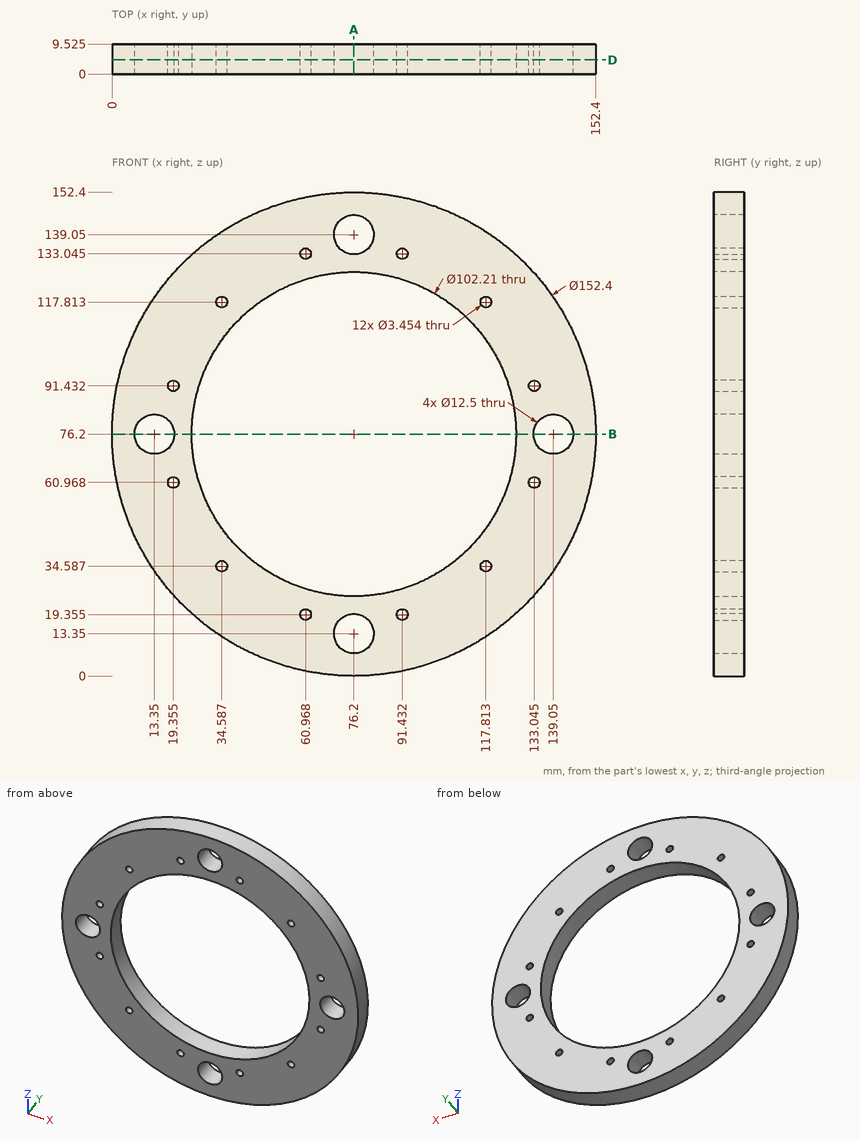
The drawing under review shows one solid part. Ordinate dimensions are in mm from its lowest x, y, z. Round coordinates to 2 decimals unless told otherwise and drop trailing zeros. Write each loop counter-clockwise with the first axis right and the second up, starting at its lowest first coordinate (ties: lowest second). Pieces come first, ordered by that corner, then holes. Notation, with made-up numbers: M 25,-16 L 66,-16 A31 cw 66,8 Z; hole C 16.5,9.5 d2. An arc over 180 degrees is marked long. One line per item, written item: value. Start each with the question number.
(1) We need section A-A (x = 76.2). Give the boundary of the cut face in (y, z) (1 decimal), and give its area (3 significant figures).
(2) Insertion check: pin 1 (1.5 mm diameter, centred on x = 119.5, y = 6.5, fed in from +Z); pin 2 (1 mm diameter, centred on x = 17, y = 5.5, fed in from +Z); pin 3 (5 mm diameter, centred on x = 57.5, y = 5, fed in from +Z). Each pin has a flat end and moves straight along its axis. Give the tip position at first contact, or say it passes through.
(3) We need section D-D (y = 4.5). Count the separate pieces of the cut face and the enclosed holes in it, and give its area (3 significant figures).
(4) Wall thickness on line 1 (X direction, y = 3.25, z = 76.2) (1 decimal); line 2 (X direction, y = 1.25, z = 71) (1 decimal); line 3 (Z direction, x = 81.5, y = 3.5) (1 decimal): over which ranges is each line inside the solid? List them lowest first.
(5) We need section B-B (z = 76.2). Give the boundary of the cut face in (x, y) (1 decimal), and give its area (3 significant figures).
Result:
1. outline: M 0,0 L 9.5,0 L 9.5,7.1 L 0,7.1 Z; M 0,19.6 L 9.5,19.6 L 9.5,25.1 L 0,25.1 Z; M 0,127.3 L 9.5,127.3 L 9.5,132.8 L 0,132.8 Z; M 0,145.3 L 9.5,145.3 L 9.5,152.4 L 0,152.4 Z
1. area: 240 mm²
2. pin 1: z = 139.41
2. pin 2: z = 124.79
2. pin 3: z = 150.66
3. separate pieces: 1
3. enclosed holes: 17
3. area: 9,430 mm²
4. line 1: 0 to 7.1, 19.6 to 25.1, 127.3 to 132.8, 145.3 to 152.4
4. line 2: 0.2 to 9.9, 16.8 to 25.4, 127 to 135.6, 142.5 to 152.2
4. line 3: 0.2 to 10, 16.7 to 25.4, 127 to 135.7, 142.4 to 152.2
5. outline: M 0,0 L 7.1,0 L 7.1,9.5 L 0,9.5 Z; M 19.6,0 L 25.1,0 L 25.1,9.5 L 19.6,9.5 Z; M 127.3,0 L 132.8,0 L 132.8,9.5 L 127.3,9.5 Z; M 145.3,0 L 152.4,0 L 152.4,9.5 L 145.3,9.5 Z
5. area: 240 mm²
